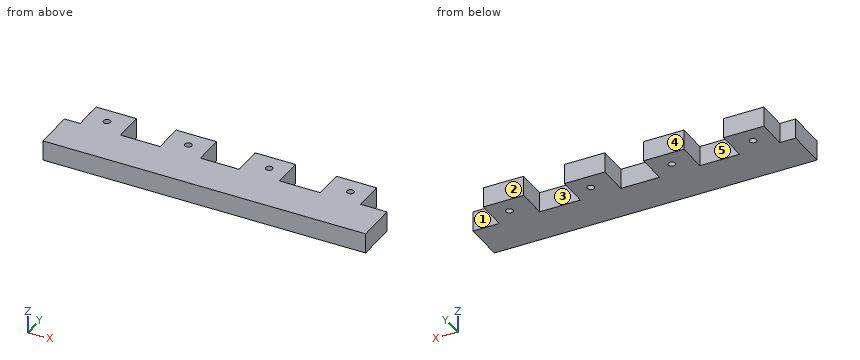
from build123d import *

# Parameters (mm, degrees)
SKETCH2_W           = 12.7
SKETCH2_H           = 9.525
SKETCH2_W_2         = 101.6
SKETCH2_H_2         = 12.7
BOSS_EXTRUDE1_DEPTH = 6.35
SKETCH1_R           = 1.0795
CUT_EXTRUDE2_DEPTH  = 7.35


with BuildPart() as part:
    # Sketch2 → Boss-Extrude1 (new body)
    with BuildSketch(Plane.XY):
        with Locations((11.316373708, 17.4625)):
            Rectangle(SKETCH2_W, SKETCH2_H)
        with Locations((50.8, 6.35)):
            Rectangle(SKETCH2_W_2, SKETCH2_H_2)
        with Locations((36.507855344, 17.4625)):
            Rectangle(SKETCH2_W, SKETCH2_H)
        with Locations((61.401212936, 17.4625)):
            Rectangle(SKETCH2_W, SKETCH2_H)
        with Locations((86.95048554, 17.4625)):
            Rectangle(SKETCH2_W, SKETCH2_H)
    extrude(amount=BOSS_EXTRUDE1_DEPTH)

    # Sketch1 → Cut-Extrude2 (cut, through all)
    with BuildSketch(Plane.XY):
        with Locations((87.798679551, 17.058161716)):
            Circle(SKETCH1_R)
        with Locations((62.206189969, 17.058161716)):
            Circle(SKETCH1_R)
        with Locations((36.698679643, 17.058161716)):
            Circle(SKETCH1_R)
        with Locations((11.106190061, 17.058161716)):
            Circle(SKETCH1_R)
        with Locations((31.326093812, 115.3905236)):
            Circle(SKETCH1_R)
        with Locations((56.918583394, 115.3905236)):
            Circle(SKETCH1_R)
        with Locations((82.42609372, 115.3905236)):
            Circle(SKETCH1_R)
        with Locations((108.018583302, 115.3905236)):
            Circle(SKETCH1_R)
    extrude(amount=CUT_EXTRUDE2_DEPTH, mode=Mode.SUBTRACT)


solid = part.part
CAD build for the part. Positions are in the model's coordinates, mm. Face numbers are marked on the shaded views. A direction names the side the tool comes from. Round coordinates to 2 decimals unless told otherwise and drop trailing zeros. Loops run counter-clockwise (first coordinate to the right, second up) from the corner with the lowest first, then second, coordinate; pieces in that order, holes last.
(1) Cut at C-C (x = 71). Give the cut face in (y, z), plus the area to 3 significant figures.
(2) Two-plate mould, pull along X, no slides. Class the marked faces 4 and 5: +X half, -X half, draft (parallel to the pull), parting line (faces both ways), or undercut.
(3) Which spindle directions (+Z, -Z, +X, -X, +Y, -Y) get a long thin tool onto all of the face, cutting with end or side? Do the marked faces 1, 2 and 3. Say none if no direction does.
(4) Cut at B-B (z = 4). Give the cut face in (x, y) (1 decimal), plus the area to 3 significant figures.
(5) Cut at A-A (y = 14.5). Give the cut face in (x, z), plus the area to 3 significant figures.
(6) Drop flat-ended pins along their axis: pin 1 (12 mm diameter, centred on x = 57, y = 8.5, fed in from -Z); pin 2 (3 mm diameter, centred on y = 17.5, z = 3, fed in from +X); pin 3 (1.7 mm diameter, centred on x = 87.8, y = 17.06, fed in from -Z); pin 4 (3 mm diameter, centred on x = 21.5, z = 4.5, fed in from +Y). Give the stop position or say it passes through.
(7) Wall check: line 1 along X through (y, z) = (12.75, 2.25); line 2 along Y through (x, z) = (46.5, 2). Give the ranges that are in metal, low to high.
Findings below:
1. outline: (0, 0) - (12.7, 0) - (12.7, 6.35) - (0, 6.35) - close
1. area: 80.6 mm2
2. face 4: draft
2. face 5: undercut
3. face 1: +Z, -Z, +X, +Y
3. face 2: +Z, -Z, +X, -X, +Y
3. face 3: +Z, -Z, +Y
4. outline: (0, 0) - (101.6, 0) - (101.6, 12.7) - (93.3, 12.7) - (93.3, 22.2) - (80.6, 22.2) - (80.6, 12.7) - (67.8, 12.7) - (67.8, 22.2) - (55.1, 22.2) - (55.1, 12.7) - (42.9, 12.7) - (42.9, 22.2) - (30.2, 22.2) - (30.2, 12.7) - (17.7, 12.7) - (17.7, 22.2) - (5, 22.2) - (5, 12.7) - (0, 12.7) - close; hole circle Ø2.2 at (11.1, 17.1); hole circle Ø2.2 at (36.7, 17.1); hole circle Ø2.2 at (62.2, 17.1); hole circle Ø2.2 at (87.8, 17.1)
4. area: 1,760 mm2
5. outline: (4.97, 0) - (17.67, 0) - (17.67, 6.35) - (4.97, 6.35) - close; (30.16, 0) - (42.86, 0) - (42.86, 6.35) - (30.16, 6.35) - close; (55.05, 0) - (67.75, 0) - (67.75, 6.35) - (55.05, 6.35) - close; (80.6, 0) - (93.3, 0) - (93.3, 6.35) - (80.6, 6.35) - close
5. area: 323 mm2
6. pin 1: stops at z = 0
6. pin 2: stops at x = 93.3
6. pin 3: passes through
6. pin 4: stops at y = 12.7
7. line 1: x = 4.97 to 17.67, 30.16 to 42.86, 55.05 to 67.75, 80.6 to 93.3
7. line 2: y = 0 to 12.7
